from build123d import *

# Parameters (mm, degrees)
SKETCH1_R                = 4
BOSS_EXTRUDE1_DEPTH      = 15
BOSS_EXTRUDE2_DEPTH      = 22
BOSS_EXTRUDE2_DEPTH_BACK = 22
SKETCH3_R                = 20
SKETCH4_R                = 10
CUT_EXTRUDE1_DEPTH       = 94.766915104
SKETCH5_R                = 4
BOSS_EXTRUDE3_DEPTH      = 2
FILLET2_R                = 2


with BuildPart() as part:
    # Sketch1 → Boss-Extrude1 (new body)
    with BuildSketch(Plane(origin=(0, 0, 0), x_dir=(1, 0, 0), z_dir=(0, 1, 0))):
        with BuildLine():
            Line((-52.5, 20), (52.5, 20))
            ThreePointArc((52.5, 20), (72.5, 0), (52.5, -20))
            Line((52.5, -20), (-52.5, -20))
            Line((-52.5, -20), (-52.5, 20))
        make_face()
        with Locations(Location((17.5, 0, 0), (0, 0, 270))):
            Circle(SKETCH1_R, mode=Mode.SUBTRACT)
        with Locations(Location((52.5, 0, 0), (0, 0, 270))):
            Circle(SKETCH1_R, mode=Mode.SUBTRACT)
    extrude(amount=BOSS_EXTRUDE1_DEPTH)

    # Sketch3 → Boss-Extrude2 (add, two sides: drawn at the far end of the back side and taken through both)
    with BuildSketch(Plane.XY.offset(-BOSS_EXTRUDE2_DEPTH_BACK)):
        with Locations((-52.411592251, 19.999804601)):
            Circle(SKETCH3_R)
    extrude(amount=BOSS_EXTRUDE2_DEPTH + BOSS_EXTRUDE2_DEPTH_BACK)

    # Sketch4 → Cut-Extrude1 (cut, through all)
    with BuildSketch(Plane.XY.offset(22)):
        with Locations((-52.411592251, 19.999804601)):
            Circle(SKETCH4_R)
    extrude(amount=-CUT_EXTRUDE1_DEPTH, mode=Mode.SUBTRACT)

    # Sketch5 → Boss-Extrude3 (add)
    with BuildSketch(Plane(origin=(0, 15, 0), x_dir=(1, 0, 0), z_dir=(0, 1, 0))):
        with BuildLine():
            Line((17.5, 15), (52.5, 15))
            ThreePointArc((52.5, 15), (67.5, 0), (52.5, -15))
            Line((52.5, -15), (17.5, -15))
            ThreePointArc((17.5, -15), (2.5, 0), (17.5, 15))
        make_face()
        with Locations(Location((17.5, 0, 0), (0, 0, 270))):
            Circle(SKETCH5_R, mode=Mode.SUBTRACT)
        with Locations(Location((52.5, 0, 0), (0, 0, 270))):
            Circle(SKETCH5_R, mode=Mode.SUBTRACT)
    extrude(amount=BOSS_EXTRUDE3_DEPTH)

    # Fillet2
    fillet2_edges = [part.edges().sort_by_distance(p)[0] for p in [
        (-33.046625069, 15, 0),
    ]]
    fillet(fillet2_edges, radius=FILLET2_R)


solid = part.part
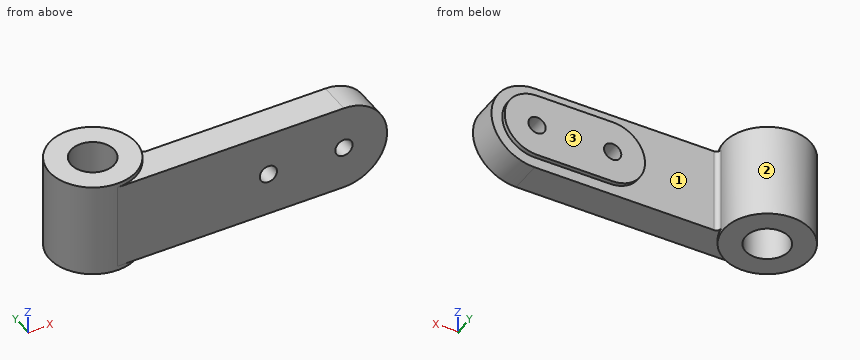
For this review, take the finished solid that the model builds, in its own axes (mm). Face numbers are marked on the shaded views. Give positions to 0.01 mm unless a question says otherwise; leave off trailing zeros. Loops run counter-clockwise (first coordinate to the right, second up) from the corner with the lowest first, then second, coordinate; pieces in that order, holes last. Notation, with made-up numbers: (43.25, -30) -> (89.25, -30) arc R28 cw to (89.25, 6) -> close; hole circle Ø4 at (86.25, 86). An arc over 180 degrees is marked (long way). One line per question, with ' | ' between items.
1) The part is to be moulded in two halves that separate along X. For the marked faces 1, 2 and 3, say which applies: +X half, -X half, draft (parallel to the pull), parting line (faces both ways), or undercut.
Resolved:
face 1: undercut | face 2: parting line | face 3: draft
2) We need section A-A (z = -2). Write out the cut boundary in (x, y).
Resolved:
outline: (-52.32, 0) -> (14.04, 0) -> (14.04, 17) -> (2.63, 17) -> (2.63, 15) -> (-30.62, 15) arc R2 cw to (-32.6, 17.27) arc R20 ccw (long way) to start; (20.96, 0) -> (49.04, 0) -> (49.04, 17) -> (20.96, 17) -> close; (55.96, 0) -> (72.4, 0) -> (72.4, 15) -> (67.37, 15) -> (67.37, 17) -> (55.96, 17) -> close; hole circle Ø20 at (-52.41, 20)
3) To check wall thickness, follow probe 1 along X at (y, z) = (25, 4.5); probe 2 along X at (y, z) = (11.5, -9.5); probe 3 along Y at (x, z) = (-47, 9.5). State the ranges of each line that lie inside material, in increasing order.
Resolved:
probe 1: x = -71.78 to -61.07, -43.75 to -33.05 | probe 2: x = -70.52 to -57.68, -47.14 to 70.1 | probe 3: y = 0 to 11.59, 28.41 to 39.25
4) We need section C-C (z = -13.5). Write out the cut boundary in (x, y), plus the area to 3 significant figures.
Resolved:
outline: (-52.32, 0) -> (67.26, 0) -> (67.26, 15) -> (59.04, 15) -> (59.04, 17) -> (10.96, 17) -> (10.96, 15) -> (-30.62, 15) arc R2 cw to (-32.6, 17.27) arc R20 ccw (long way) to start; hole circle Ø20 at (-52.41, 20) | area: 2,620 mm2
5) We need section D-D (x = -15). Write out the cut boundary in (y, z), plus the area to 3 significant figures.
Resolved:
outline: (0, -20) -> (15, -20) -> (15, 20) -> (0, 20) -> close | area: 600 mm2
6) Insertion check: pin 1 Ø1.5 at (x, z) = (16, 10) entering from +Y; pin 2 Ø4 at (y, z) = (31, 12.5) entering from +X; pin 3 Ø19 at (x, y) = (10.5, 12) entering from -Z. Each pin has a flat end and moves straight along its axis. Give the tip position at first contact, or say it passes through.
Resolved:
pin 1: stops at y = 17 | pin 2: stops at x = -34.55 | pin 3: stops at z = -20
7) We need section B-B (y = 5). Write out the cut boundary in (x, z), plus the area to 3 significant figures.
Resolved:
outline: (-65.64, -22) -> (-39.18, -22) -> (-39.18, -20) -> (52.5, -20) arc R20 ccw to (52.5, 20) -> (-39.18, 20) -> (-39.18, 22) -> (-65.64, 22) -> close; hole circle Ø8 at (17.5, 0); hole circle Ø8 at (52.5, 0) | area: 5,360 mm2
